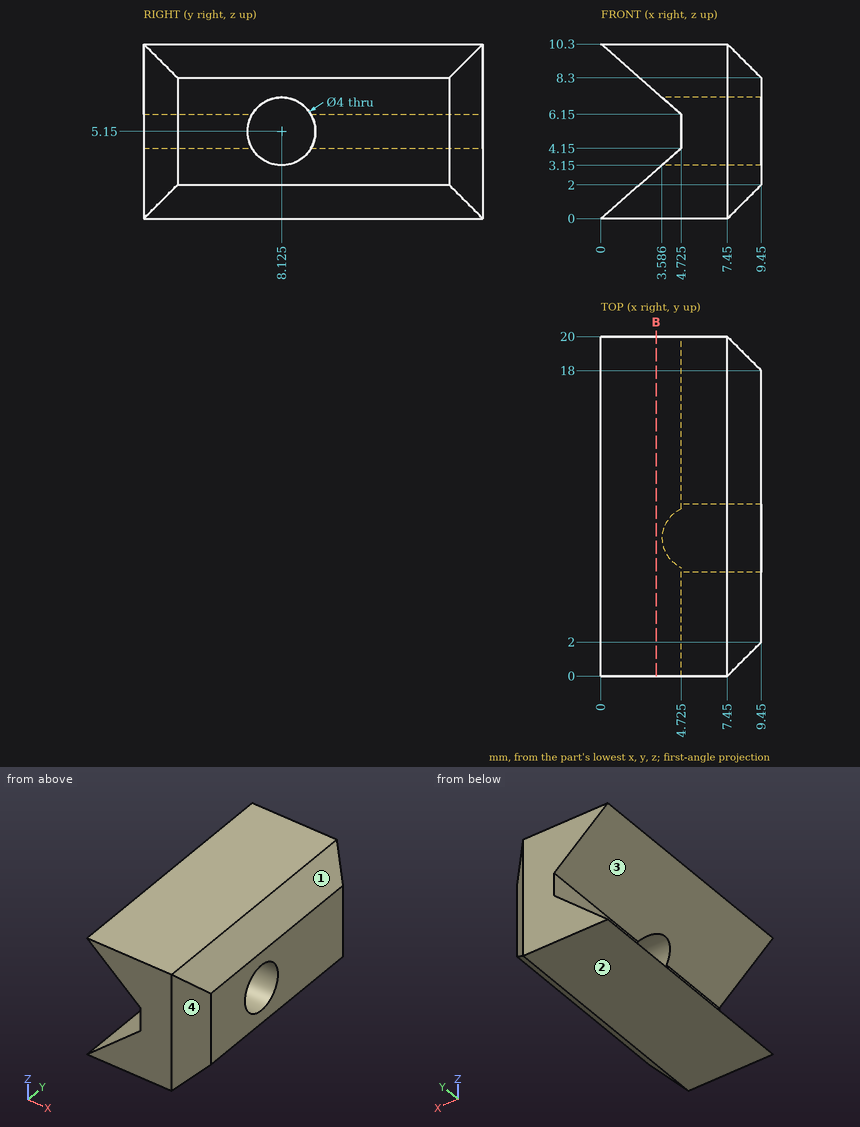
Could you check a few things on this drawing? It's one solid part, dimensions in mm from its lowest x, y, z. Round coordinates to 2 decimals unless told otherwise and drop trailing zeros. Write each loop counter-clockwise with the first axis right and the second up, starting at its lowest first coordinate (ties: lowest second). Pieces come first, ordered by that corner, then holes.
Q1. If we section it at B-B on x = 3.25: Write out the boundary of the cut face in (y, z) (1 decimal), plus the area to 3 significant figures.
Q2. Please list where these lines run through material, in increasing order: probe 1 along Y at (x, z) = (6, 5.15) (1 decimal); probe 2 along Z at (x, y) = (2.75, 12.25) (1 decimal); probe 3 along Z at (x, y) = (8.75, 9.75) (1 decimal).
Q3. If we mould it in two halves opening along Z, with no side actions, what happens to the marked faces 1, 2, 3 and 4? For each: +Z half, -Z half, draft (parallel to the pull), parting line (faces both ways), or undercut.
Q4. Will these pins go through, and if not, where does the flat tip stop? P1, Ø0.6, axis at y = 14, z = 5, coming from the -X side (3 decimals); P2, Ø5, axis at y = 10.5, z = 5.5, coming from the -X side; P3, Ø5, axis at x = 8.5, y = 14, coming from the +Z side.
Answer below:
1. outline: (0, 0) - (20, 0) - (20, 2.9) - (0, 2.9) - close; (0, 7.4) - (20, 7.4) - (20, 10.3) - (0, 10.3) - close
1. area: 114 mm2
2. probe 1: y = 0 to 6.1, 10.1 to 20
2. probe 2: z = 0 to 2.4, 7.9 to 10.3
2. probe 3: z = 1.3 to 4, 6.3 to 9
3. face 1: +Z half
3. face 2: -Z half
3. face 3: undercut
3. face 4: draft
4. P1: stops at x = 4.725
4. P2: stops at x = 2.62
4. P3: stops at z = 10.3
